Design review of the part built by this model. Coordinates are the model's own, in mm. A direction names the side the tool comes from. Coordinates: 2 decimals unless noted, no trailing zeros. Write each loop counter-clockwise with the first axis right and the second up, starting at its lowest first coordinate (ties: lowest second). Pieces come first, ordered by that corner, then holes.
Q1. Take a section at A-A (y = -10). Give the boundary of the cut face in (x, z) (3 decimals).
Q2. Machinability: for faces 4 (the cylindrical face through (-17.524, 2.817, 0.176)), 5 (the cylindrical face through (7.708, -17.867, 0.572)), 6 (the flat face through (-10, -12.7, 0)), 7 (the flat face through (-8, -14.155, 0)), which of the approach directions +Z, -Z, +X, -X, +Y, -Y give a long, thin tool a straight path to every point of the face, cutting with its end or side? Answer none if there is none.
Q3. Insertion check: pin 1 (1.3 mm diameter, centred on x = 9.5, z = 0.5, fed in from +Y); pin 2 (3 mm diameter, centred on x = -9.5, y = -12.5, fed in from +Z) (3 decimals); pin 3 (8 mm diameter, centred on y = -11.5, z = 1.5, fed in from -X). Each pin has a flat end and moves straight along its axis. Give the tip position at first contact, or say it passes through.
Q4. Mouldability with a two-part tool opening along Y and no side actions: class faces 1 (the flat face through (-11, -17.457, 0)), 2 (the flat face through (0, 3, -8.001)), 3 (the flat face through (8.2, 12.7, -2.5)) as pulls with the +Y half, pulls with the -Y half, needs draft (parallel to the pull), parting line crosses it, or undercut.
Q5. For probe 1 along X at (y, z) = (0.5, 0); probe 2 along X at (y, z) = (0.5, 1.5); probe 3 along Y at (x, z) = (14.5, 4.5), list the stretches that pass through material, from the lowest coordinate up.
```python
from build123d import *

# Parameters (mm, degrees)
BOSS_EXTRUDE1_DEPTH = 6.35
SKETCH2_R           = 6.35
BOSS_EXTRUDE2_DEPTH = 6.35
BOSS_EXTRUDE2_TAPER = 3
SKETCH3_R           = 4.699
BOSS_EXTRUDE3_DEPTH = 0.889
LPATTERN1_COUNT     = 2
LPATTERN1_PITCH     = 19.05
FILLET1_R           = 0.635
SKETCH5_R           = 2.1082
CUT_EXTRUDE1_DEPTH  = 25.4


with BuildPart() as part:
    # Sketch1 → Boss-Extrude1 (new body)
    with BuildSketch(Plane(origin=(0, 0, 0), x_dir=(1, 0, 0), z_dir=(0, 1, 0))):
        with BuildLine():
            Line((-9.525, 8.001), (9.525, 8.001))
            ThreePointArc((9.525, 8.001), (17.526, 0), (9.525, -8.001))
            Line((9.525, -8.001), (-9.525, -8.001))
            ThreePointArc((-9.525, -8.001), (-17.526, 0), (-9.525, 8.001))
        make_face()
    extrude(amount=BOSS_EXTRUDE1_DEPTH)

    # Sketch2 → Boss-Extrude2 (add)
    with BuildSketch(Plane(origin=(0, 6.35, 0), x_dir=(1, 0, 0), z_dir=(0, 1, 0))):
        with Locations((-9.525, 0)):
            Circle(SKETCH2_R)
        with Locations((9.525, 0)):
            Circle(SKETCH2_R)
    extrude(amount=BOSS_EXTRUDE2_DEPTH, taper=BOSS_EXTRUDE2_TAPER)

    # Sketch3 → Boss-Extrude3 (add)
    with BuildSketch(Plane.XZ):
        with Locations((-9.525, 0)):
            Circle(SKETCH3_R)
        with Locations((9.525, 0)):
            Circle(SKETCH3_R)
    extrude(amount=BOSS_EXTRUDE3_DEPTH)

    # Sketch4 → Revolve1 (revolve)
    with BuildSketch(Plane.XY):
        Polygon((9.525, -0.889), (9.525, -18.288), (7.62, -18.288), (7.62, -17.456876592), (8.382, -17.456876592), (8.382, -14.154876592), (6.35, -14.154876592), (6.35, -0.889), align=None)
    revolve1 = revolve(axis=Axis((9.525, -0.889, 0), (0, 1, 0)))

    # LPattern1: Revolve1 ×2
    with Locations(*[(-i * LPATTERN1_PITCH, 0, 0) for i in range(1, LPATTERN1_COUNT)]):
        add(revolve1)

    # Fillet1
    fillet1_edges = [part.edges().sort_by_distance(p)[0] for p in [
        (17.526, 6.35, 0),
        (0, 6.35, -8.001),
        (-15.542210602, 12.7, 0),
        (3.507789398, 12.7, 0),
        (-17.526, 6.35, 0),
        (0, 6.35, 8.001),
    ]]
    fillet(fillet1_edges, radius=FILLET1_R)

    # Sketch5 → Cut-Extrude1 (cut)
    with BuildSketch(Plane(origin=(0, 12.7, 0), x_dir=(1, 0, 0), z_dir=(0, 1, 0))):
        with Locations((-9.525, 0)):
            Circle(SKETCH5_R)
        with Locations((9.525, 0)):
            Circle(SKETCH5_R)
    extrude(amount=-CUT_EXTRUDE1_DEPTH, mode=Mode.SUBTRACT)

    # Sketch6 → flare (revolve, cut)
    with BuildSketch(Plane.XY):
        Polygon((6.409091305, 15.24), (7.4168, 9.525), (8.424508695, 15.24), align=None)
    flare = revolve(axis=Axis((9.525, -12.7, 0), (0, 1, 0)), mode=Mode.SUBTRACT)

    # Mirror1: flare across plane
    add(flare.mirror(Plane(origin=(0, 0, 0), x_dir=(0, 0, 1), z_dir=(1, 0, 0))), mode=Mode.SUBTRACT)


solid = part.part
```
Response:
1. outline: circle Ø6.35 at (-9.525, 0); circle Ø6.35 at (9.525, 0); hole circle Ø4.216 at (-9.525, 0); hole circle Ø4.216 at (9.525, 0)
2. face 4: -X, +Y, -Y
2. face 5: -Y
2. face 6: +Y
2. face 7: none
3. pin 1: stops at y = -12.7
3. pin 2: stops at z = 3.175
3. pin 3: stops at x = -12.7
4. face 1: undercut
4. face 2: needs draft
4. face 3: pulls with the +Y half
5. probe 1: x = -17.53 to -11.63, -7.42 to 7.42, 11.63 to 17.53
5. probe 2: x = -17.38 to -11.01, -8.04 to 8.04, 11.01 to 17.38
5. probe 3: y = 0 to 6.35
